For this review, take the finished solid that the model builds, in its own axes (mm). Face numbers are marked on the shaded views. Give positions to 0.01 mm unless a question says otherwise; leave off trailing zeros. Write each loop counter-clockwise with the first axis right and the second up, starting at its lowest first coordinate (ties: lowest second). Pieces come first, ordered by that corner, then holes.
Q1. Insertion check: P1, Ø2.5, axis at x = 31, z = -2, coming from the +Y side. The pin has a flat end and moves straight along its axis. Give the tip position at first contact, or say it passes through.
Q2. We need section C-C (z = -0.2). Give the number of separate pieces and of enclosed holes in the cut face, then the cut area to 3 significant figures.
Q3. Mouldability with a two-part tool opening along Z and no side actions: class the marked faces 1, 2, 3 and 4 as released by +Z, released by -Z, zero draft, split by the parting line, or undercut.
Q4. We need section B-B (y = 7.5). Write out the cut boundary in (x, z), then the cut area to 3 significant figures.
Q5. We need section A-A (x = 20). Write out the cut boundary in (y, z).
Q6. For line 1 (Z direction, x = -30, y = 4.75); line 2 (X direction, y = 8.5, z = 6); line 3 (Y direction, x = -20, z = -4), list the stretches that pass through material, from the lowest coordinate up.
Q7. We need section D-D (z = 6). Write out the cut boundary in (x, y).
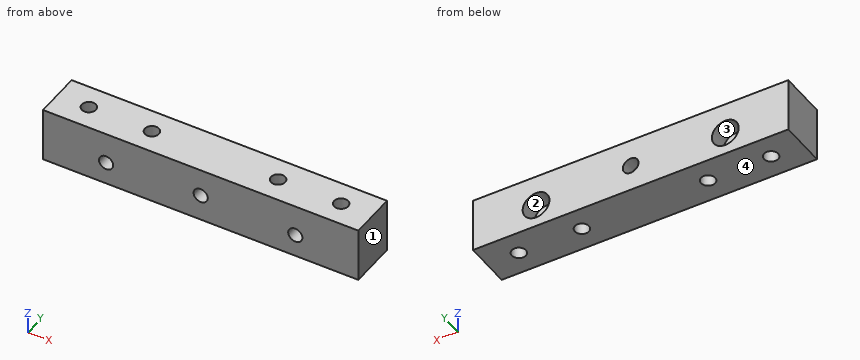
```python
from build123d import *

# Parameters (mm, degrees)
SKETCH1_W                               = 100
SKETCH1_H                               = 17.228
BOSS_EXTRUDE1_DEPTH                     = 15
CBORE_FOR_M5_HEX_HEAD_BOLT1_D           = 4.5
CBORE_FOR_M5_HEX_HEAD_BOLT1_CBORE_D     = 8.5
CBORE_FOR_M5_HEX_HEAD_BOLT1_CBORE_DEPTH = 6
M4_CLEARANCE_HOLE1_D                    = 4.5
CBORE_FOR_M5_HEX_HEAD_BOLT2_D           = 4.5
CBORE_FOR_M5_HEX_HEAD_BOLT2_CBORE_D     = 5
CBORE_FOR_M5_HEX_HEAD_BOLT2_CBORE_DEPTH = 4.2


with BuildPart() as part:
    # Sketch1 → Boss-Extrude1 (new body)
    with BuildSketch(Plane(origin=(0, 0, 0), x_dir=(1, 0, 0), z_dir=(0, 1, 0))):
        Rectangle(SKETCH1_W, SKETCH1_H)
    extrude(amount=BOSS_EXTRUDE1_DEPTH)

    # CBORE for M5 Hex Head Bolt1 (through all)
    with Locations(Plane(origin=(0, 15, 0), x_dir=(1, 0, 0), z_dir=(0, 1, 0))):
        with Locations((-30, 1.386), (30, 1.386)):
            CounterBoreHole(CBORE_FOR_M5_HEX_HEAD_BOLT1_D / 2, CBORE_FOR_M5_HEX_HEAD_BOLT1_CBORE_D / 2, CBORE_FOR_M5_HEX_HEAD_BOLT1_CBORE_DEPTH)

    # M4 Clearance Hole1 (through all)
    with Locations(Plane.XY.offset(8.614)):
        with Locations((-20, 7.5), (20, 7.5), (-40, 7.5), (40, 7.5)):
            Hole(M4_CLEARANCE_HOLE1_D / 2)

    # CBORE for M5 Hex Head Bolt2 (through all)
    with Locations(Plane(origin=(0, 15, 0), x_dir=(1, 0, 0), z_dir=(0, 1, 0))):
        with Locations((0, 0.2)):
            CounterBoreHole(CBORE_FOR_M5_HEX_HEAD_BOLT2_D / 2, CBORE_FOR_M5_HEX_HEAD_BOLT2_CBORE_D / 2, CBORE_FOR_M5_HEX_HEAD_BOLT2_CBORE_DEPTH)


solid = part.part
```
Computed:
1. P1: stops at y = 9
2. separate pieces: 4
2. enclosed holes: 4
2. area: 1,200 mm2
3. face 1: zero draft
3. face 2: undercut
3. face 3: undercut
3. face 4: released by -Z
4. outline: (-50, -8.61) - (-42.25, -8.61) - (-42.25, 8.61) - (-50, 8.61) - close; (-37.75, -8.61) - (-22.25, -8.61) - (-22.25, 8.61) - (-37.75, 8.61) - close; (-17.75, -8.61) - (17.75, -8.61) - (17.75, 8.61) - (-17.75, 8.61) - close; (22.25, -8.61) - (37.75, -8.61) - (37.75, 8.61) - (22.25, 8.61) - close; (42.25, -8.61) - (50, -8.61) - (50, 8.61) - (42.25, 8.61) - close; hole circle Ø4.5 at (-30, -1.39); hole circle Ø4.5 at (0, -0.2); hole circle Ø4.5 at (30, -1.39)
4. area: 1,360 mm2
5. outline: (0, -8.61) - (5.25, -8.61) - (5.25, 8.61) - (0, 8.61) - close; (9.75, -8.61) - (15, -8.61) - (15, 8.61) - (9.75, 8.61) - close
6. line 1: z = -8.61 to -3.64, 0.86 to 8.61
6. line 2: x = -50 to -42.02, -37.98 to -22.02, -17.98 to 17.98, 22.02 to 37.98, 42.02 to 50
6. line 3: y = 0 to 5.25, 9.75 to 15
7. outline: (-50, 0) - (50, 0) - (50, 15) - (-50, 15) - close; hole circle Ø4.5 at (-40, 7.5); hole circle Ø4.5 at (-20, 7.5); hole circle Ø4.5 at (20, 7.5); hole circle Ø4.5 at (40, 7.5)
